CAD build for the part. Positions are in the model's coordinates, mm. A direction names the side the tool comes from. Round coordinates to 2 decimals unless told otherwise and drop trailing zeros. Order: outer loops, then holes, each group sorted by start corner. A loop starts at its lowest first (then second) coordinate and runs counter-clockwise, first axis right, second up. Notation, with made-up numbers: M 53.25,-4.75 L 104.25,-4.75 A7 ccw 104.25,1.25 Z; hole C 18.25,59 d11. An arc over 180 degrees is marked long. Put each result on its own line as item: value.
```python
from build123d import *

# Parameters (mm, degrees)
SKETCH1_R           = 15
SKETCH1_R_2         = 12.5
BOSS_EXTRUDE1_DEPTH = 85
CUT_EXTRUDE1_START  = -1.375
SKETCH2_R           = 15
SKETCH2_R_2         = 14
CUT_EXTRUDE1_DEPTH  = 1.375
CHAMFER1_SIZE       = 1.25
CHAMFER2_SIZE       = 1


with BuildPart() as part:
    # Sketch1 → Boss-Extrude1 (new body)
    with BuildSketch(Plane(origin=(0, 0, 0), x_dir=(1, 0, 0), z_dir=(0, 1, 0))):
        with Locations(Location((0, 0, 0), (0, 0, 270))):
            Circle(SKETCH1_R)
        with Locations(Location((0, 0, 0), (0, 0, 270))):
            Circle(SKETCH1_R_2, mode=Mode.SUBTRACT)
    extrude(amount=BOSS_EXTRUDE1_DEPTH)

    # Sketch2 → Cut-Extrude1 (cut)
    with BuildSketch(Plane(origin=(0, 81.875, 0), x_dir=(1, 0, 0), z_dir=(0, 1, 0)).offset(CUT_EXTRUDE1_START)):
        with Locations(Location((0, 0, 0), (0, 0, 270))):
            Circle(SKETCH2_R)
        with Locations(Location((0, 0, 0), (0, 0, 270))):
            Circle(SKETCH2_R_2, mode=Mode.SUBTRACT)
    cut_extrude1 = extrude(amount=CUT_EXTRUDE1_DEPTH, mode=Mode.SUBTRACT)

    # Mirror1: Cut-Extrude1 across plane
    add(cut_extrude1.mirror(Plane.ZX.offset(42.5)), mode=Mode.SUBTRACT)

    # Chamfer1
    chamfer1_edges = [part.edges().sort_by_distance(p)[0] for p in [
        (0, 0, -12.5),
        (0, 85, -12.5),
    ]]
    chamfer(chamfer1_edges, length=CHAMFER1_SIZE)

    # Chamfer2
    chamfer2_edges = [part.edges().sort_by_distance(p)[0] for p in [
        (0, 0, -15),
        (0, 85, -15),
    ]]
    chamfer(chamfer2_edges, length=CHAMFER2_SIZE)


solid = part.part
```
Item 1: Band-saw the part on C-C on y = 52. Give the cut face in (x, z), and give its area (3 significant figures).
Answers below:
outline: C 0,0 d30; hole C 0,0 d25
area: 216 mm²
Item 2: Pin check, flat tips, straight feed: P1, Ø1, axis at x = -5, z = -11, coming from the +Y side; P2, Ø15, axis at x = 0, z = 0, coming from the +Y side; P3, Ø3, axis at x = -11, y = 18.5, coming from the +Z side; P4, Ø1.5, axis at x = -1, y = 14, coming from the +Z side. Stop position of each tip, or through.
Answers below:
P1: y = 83.83
P2: through
P3: z = 11.61
P4: z = 15
Item 3: Tool access for faces 3 (the cylindrical face through (0.66, 2.048, -14.985)), 4 (the cylindrical face through (-13.67, 81.18, -3.03)): list every direction of +Z, -Z, +X, -X, +Y, -Y with a clear straight run to the whole face (end or side of a thin tool).
Answers below:
face 3: +Y, -Y
face 4: none
Item 4: Mould opens along Z. For faces 1 (the cylindrical face through (3.755, 41.922, 11.923)), 2 (the cylindrical face through (-13.67, 3.82, -3.03)) say: pulls with the +Z half, pulls with the -Z half, needs draft (parallel to the pull), parting line crosses it, or undercut.
Answers below:
face 1: undercut
face 2: parting line crosses it
Item 5: Probe line 1 along X through (y, z) = (38, 0); line 2 along Y through (x, z) = (13.5, 4.75) (3 decimals); line 3 along Z through (x, y) = (-11.5, 70). List the from-to ranges inside material, lowest first. Write a range as [from, to].
Answers below:
line 1: [-15, -12.5], [12.5, 15]
line 2: [0.311, 3.125], [4.5, 80.5], [81.875, 84.689]
line 3: [-9.63, -4.9], [4.9, 9.63]
